Build history of the part. All positions in model axes, mm. A direction names the side the tool comes from. Round coordinates to 2 decimals unless told otherwise and drop trailing zeros. Write each loop counter-clockwise with the first axis right and the second up, starting at its lowest first coordinate (ties: lowest second). Pieces come first, ordered by that corner, then holes. Notation, with made-up numbers: M 79.5,25.5 L 109.5,25.5 A14 ccw 109.5,37.5 Z; hole C -35,89 d9. An arc over 180 degrees is marked long. Use a Markdown table: item, result.
from build123d import *

# Parameters (mm, degrees)
SKETCH_1_W             = 150
SKETCH_1_H             = 150
EXTRUDE_1_DEPTH        = 6
SKETCH_2_R             = 42.5
CUT_EXTRUDE_1_DEPTH    = 1
CHAMFER_1_SIZE         = 5
SKETCH_4_R             = 1.5
CUT_EXTRUDE_3_DEPTH    = 10
SKETCH_5_R             = 2.85
CUT_EXTRUDE_4_DEPTH    = 3.2
SKETCH_6_R             = 1.5
CUT_EXTRUDE_5_DEPTH    = 10
SKETCH_7_R             = 2.85
CUT_EXTRUDE_6_DEPTH    = 3.2
SKETCH_8_R             = 4.5
CUT_EXTRUDE_7_DEPTH    = 10
SKETCH_9_R             = 2
CUT_EXTRUDE_8_DEPTH    = 10
SKETCH_10_R            = 1
CUT_EXTRUDE_9_DEPTH    = 10
HOLE_WIZARD_M3_1_D     = 2.5
HOLE_WIZARD_M3_1_DEPTH = 7.5
HOLE_WIZARD_M3_1_TIP   = 0.751075774
SKETCH_15_R            = 25.5
CUT_EXTRUDE_12_DEPTH   = 3
SKETCH_16_R            = 1.5
CUT_EXTRUDE_13_DEPTH   = 3
SKETCH_17_R            = 1
CUT_EXTRUDE_14_DEPTH   = 10
HOLE_WIZARD_M3_2_D     = 2.5
HOLE_WIZARD_M3_2_DEPTH = 7.5
HOLE_WIZARD_M3_2_TIP   = 0.751075774


with BuildPart() as part:
    # 草图1 → 凸台-拉伸1 (new body)
    with BuildSketch(Plane.XY):
        Rectangle(SKETCH_1_W, SKETCH_1_H)
    extrude(amount=EXTRUDE_1_DEPTH)

    # 草图2 → 切除-拉伸1 (cut)
    with BuildSketch(Plane.XY.offset(6)):
        with Locations((0, -15)):
            Circle(SKETCH_2_R)
    extrude(amount=-CUT_EXTRUDE_1_DEPTH, mode=Mode.SUBTRACT)

    # 倒角1
    chamfer_1_edges = [part.edges().sort_by_distance(p)[0] for p in [
        (-75, 75, 3),
        (75, 75, 3),
        (75, -75, 3),
        (-75, -75, 3),
    ]]
    chamfer(chamfer_1_edges, length=CHAMFER_1_SIZE)

    # 草图4 → 切除-拉伸3 (cut)
    with BuildSketch(Plane.XY.offset(6)):
        with Locations((64, 71)):
            Circle(SKETCH_4_R)
        with Locations((71, 64)):
            Circle(SKETCH_4_R)
    cut_extrude_3 = extrude(amount=-CUT_EXTRUDE_3_DEPTH, mode=Mode.SUBTRACT)

    # 草图5 → 切除-拉伸4 (cut)
    with BuildSketch(Plane.XY.offset(6)):
        with Locations((64, 71)):
            Circle(SKETCH_5_R)
        with Locations((71, 64)):
            Circle(SKETCH_5_R)
    cut_extrude_4 = extrude(amount=-CUT_EXTRUDE_4_DEPTH, mode=Mode.SUBTRACT)

    # 草图6 → 切除-拉伸5 (cut)
    with BuildSketch(Plane.XY.offset(6)):
        with Locations((-64, 71)):
            Circle(SKETCH_6_R)
        with Locations((-71, 64)):
            Circle(SKETCH_6_R)
    cut_extrude_5 = extrude(amount=-CUT_EXTRUDE_5_DEPTH, mode=Mode.SUBTRACT)

    # 草图7 → 切除-拉伸6 (cut)
    with BuildSketch(Plane.XY.offset(6)):
        with Locations((-64, 71)):
            Circle(SKETCH_7_R)
        with Locations((-71, 64)):
            Circle(SKETCH_7_R)
    cut_extrude_6 = extrude(amount=-CUT_EXTRUDE_6_DEPTH, mode=Mode.SUBTRACT)

    # 镜向1: 切除-拉伸3, 切除-拉伸4, 切除-拉伸5, 切除-拉伸6 across plane
    add(cut_extrude_3.mirror(Plane.ZX), mode=Mode.SUBTRACT)
    add(cut_extrude_4.mirror(Plane.ZX), mode=Mode.SUBTRACT)
    add(cut_extrude_5.mirror(Plane.ZX), mode=Mode.SUBTRACT)
    add(cut_extrude_6.mirror(Plane.ZX), mode=Mode.SUBTRACT)

    # 草图8 → 切除-拉伸7 (cut)
    with BuildSketch(Plane.XY.offset(5)):
        with Locations((0, -15)):
            Circle(SKETCH_8_R)
    extrude(amount=-CUT_EXTRUDE_7_DEPTH, mode=Mode.SUBTRACT)

    # 草图9 → 切除-拉伸8 (cut)
    with BuildSketch(Plane.XY.offset(5)):
        with Locations((-12, -15)):
            Circle(SKETCH_9_R)
        with Locations((12, -15)):
            Circle(SKETCH_9_R)
        with Locations((0, -27)):
            Circle(SKETCH_9_R)
        with Locations((0, -3)):
            Circle(SKETCH_9_R)
    extrude(amount=-CUT_EXTRUDE_8_DEPTH, mode=Mode.SUBTRACT)

    # 草图10 → 切除-拉伸9 (cut)
    with BuildSketch(Plane.XY.offset(5)):
        with Locations((0, 22.5)):
            Circle(SKETCH_10_R)
        with Locations((37.5, -15)):
            Circle(SKETCH_10_R)
        with Locations((0, -52.5)):
            Circle(SKETCH_10_R)
        with Locations((-37.5, -15)):
            Circle(SKETCH_10_R)
    extrude(amount=-CUT_EXTRUDE_9_DEPTH, mode=Mode.SUBTRACT)

    # M3 螺纹孔1
    with Locations(Plane.XY.offset(5)):
        with Locations((0, 22.5), (-37.5, -15), (0, -52.5), (37.5, -15)):
            Hole(HOLE_WIZARD_M3_1_D / 2, depth=HOLE_WIZARD_M3_1_DEPTH)
            with Locations((0, 0, -(HOLE_WIZARD_M3_1_DEPTH + HOLE_WIZARD_M3_1_TIP / 2))):  # 118° drill point
                Cone(0, HOLE_WIZARD_M3_1_D / 2, HOLE_WIZARD_M3_1_TIP, mode=Mode.SUBTRACT)

    # 草图15 → 切除-拉伸12 (cut)
    with BuildSketch(Plane(origin=(0, 0, 0), x_dir=(-1, 0, 0), z_dir=(0, 0, -1))):
        with Locations((41, 41)):
            Circle(SKETCH_15_R)
    extrude(amount=-CUT_EXTRUDE_12_DEPTH, mode=Mode.SUBTRACT)

    # 草图16 → 切除-拉伸13 (cut)
    with BuildSketch(Plane(origin=(0, 0, 3), x_dir=(-1, 0, 0), z_dir=(0, 0, -1))):
        with Locations((41, 41)):
            Circle(SKETCH_16_R)
        with Locations((41, 48.5)):
            Circle(SKETCH_16_R)
        with Locations((48.5, 41)):
            Circle(SKETCH_16_R)
        with Locations((41, 33.5)):
            Circle(SKETCH_16_R)
        with Locations((33.5, 41)):
            Circle(SKETCH_16_R)
        with Locations((41, 56)):
            Circle(SKETCH_16_R)
        with Locations((51.606601718, 51.606601718)):
            Circle(SKETCH_16_R)
        with Locations((56, 41)):
            Circle(SKETCH_16_R)
        with Locations((51.606601718, 30.393398282)):
            Circle(SKETCH_16_R)
        with Locations((41, 26)):
            Circle(SKETCH_16_R)
        with Locations((30.393398282, 30.393398282)):
            Circle(SKETCH_16_R)
        with Locations((26, 41)):
            Circle(SKETCH_16_R)
        with Locations((30.393398282, 51.606601718)):
            Circle(SKETCH_16_R)
    extrude(amount=-CUT_EXTRUDE_13_DEPTH, mode=Mode.SUBTRACT)

    # 草图17 → 切除-拉伸14 (cut)
    with BuildSketch(Plane.XY.offset(6)):
        with Locations((0, -61.5)):
            Circle(SKETCH_17_R)
        with Locations((0, -71)):
            Circle(SKETCH_17_R)
    extrude(amount=-CUT_EXTRUDE_14_DEPTH, mode=Mode.SUBTRACT)

    # M3 螺纹孔2
    with Locations(Plane.XY.offset(6)):
        with Locations((0, -61.5), (0, -71)):
            Hole(HOLE_WIZARD_M3_2_D / 2, depth=HOLE_WIZARD_M3_2_DEPTH)
            with Locations((0, 0, -(HOLE_WIZARD_M3_2_DEPTH + HOLE_WIZARD_M3_2_TIP / 2))):  # 118° drill point
                Cone(0, HOLE_WIZARD_M3_2_D / 2, HOLE_WIZARD_M3_2_TIP, mode=Mode.SUBTRACT)


solid = part.part
Q1. Cut at B-B on x = 12. Give the cut face in (y, z).
Response values:
| item | result |
|---|---|
| outline | M -75,0 L -17,0 L -17,5 L -55.77,5 L -55.77,6 L -75,6 Z; M -13,0 L 75,0 L 75,6 L 25.77,6 L 25.77,5 L -13,5 Z |
Q2. Drop flat-ended pins along their axis: P1, Ø3.5, axis at x = -30.39, y = 51.61, coming from the -Z side; P2, Ø4, axis at x = -71, y = 64, coming from the +Z side; P3, Ø8, axis at x = 0, y = -15, coming from the -Z side; P4, Ø4.5, axis at x = -12, y = -15, coming from the +Z side. Give the stop position or say it passes through.
Response values:
| item | result |
|---|---|
| P1 | stops at z = 3 |
| P2 | stops at z = 2.8 |
| P3 | passes through |
| P4 | stops at z = 5 |
Q3. Cut at A-A on z = 1.4. Count the separate pieces of the cut face and the enclosed holes in it, and give its area (3 significant figures).
Response values:
| item | result |
|---|---|
| separate pieces | 1 |
| enclosed holes | 20 |
| area | 20,200 mm2 |
Q4. Which spindle directions (+Z, -Z, +X, -X, +Y, -Y) get a long thin tool onto all of the face, cutting with end or side? Do faces 1 (the flat face through (-72, -73, 3)), 2 (the cylindrical face through (-65.322, 48.66, 1.479)), 3 (the cylindrical face through (-61.282, -71.856, 4.422)). Say none if no direction does.
Response values:
| item | result |
|---|---|
| face 1 | +Z, -Z, -X, -Y |
| face 2 | -Z |
| face 3 | +Z |
Q5. Drill centre lines: L1, parallel to Y at x = -64, z = 3.6; L2, parallel to Y at x = -51.5, z = 5.55; L3, parallel to Y at x = -12, z = 2.85. Where is each one in solid material? Low to high.
Response values:
| item | result |
|---|---|
| L1 | y = -75 to -73.85, -68.15 to 68.15, 73.85 to 75 |
| L2 | y = -75 to 28.9, 31.89 to 50.11, 53.1 to 75 |
| L3 | y = -75 to -17, -13 to 75 |
Q6. Two-plate mould, pull along X, no slides. Class faces 4 (the flat face through (65.2, 69.8, 2.8)), 5 (the flat face through (-72, 73, 3)), 6 (the flat face through (-1, -75, 3)): +X half, -X half, draft (parallel to the pull), parting line (faces both ways), or undercut.
Response values:
| item | result |
|---|---|
| face 4 | undercut |
| face 5 | -X half |
| face 6 | draft |
